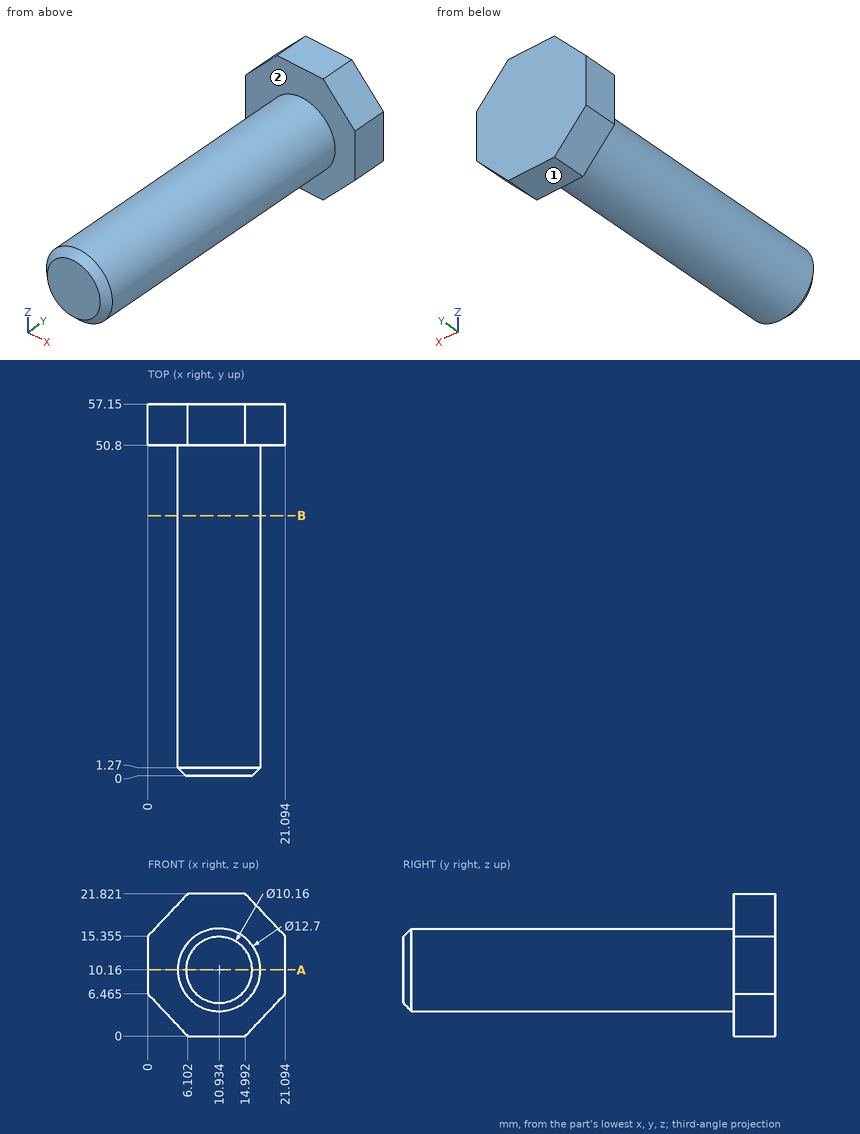
Answer from the drawing. Dimensions are ordinates in mm from the lowest x, y and z of the part. A direction names the side the tool comes from. Give positions to 0.01 mm unless a question says otherwise; leave off trailing zeros. Write each loop counter-clockwise with the first axis right and the second up, starting at its lowest first coordinate (ties: lowest second). Pieces come first, ordered by that corner, then holes.
1) Find the intervals of material crossed by L1, parallel to Y at x = 13.25, z = 16.25; L2, parallel to Z at x = 14.75, y = 35.5 (1 decimal); L3, parallel to X at y = 11, z = 10.25 (1 decimal), in increasing order.
2) Section A-A (z = 10.16) is taken. Write down the section's boundary in (x, y).
3) A tool of negligible diameter and unlimited length cuts with its end or side. For the marked faces 1 and 2, from which of +Z, -Z, +X, -X, +Y, -Y can it reach the whole face along a straight path? Write none if from no direction.
4) Given P1, Ø6, axis at x = 7, y = 26, coming from the +Z side; P2, Ø3, axis at x = 11.5, y = 32.5, coming from the +Z side; P3, Ø3, axis at y = 43, z = 8, coming from the -X side; P4, Ø8, axis at x = 11.5, z = 11.5, coming from the -Y side, each flat-ended and moving along its own axis, determine where each tip first touches the part or whether it passes through.
5) Section B-B (y = 40) is taken. Write down the section's boundary in (x, z).
Response:
1. L1: y = 50.8 to 57.15
1. L2: z = 5.1 to 15.2
1. L3: x = 4.6 to 17.3
2. outline: (0, 50.8) - (4.58, 50.8) - (4.58, 1.27) - (5.85, 0) - (16.01, 0) - (17.28, 1.27) - (17.28, 50.8) - (21.09, 50.8) - (21.09, 57.15) - (0, 57.15) - close
3. face 1: -Z, +X, -X, +Y, -Y
3. face 2: -Y
4. P1: stops at z = 16.44
4. P2: stops at z = 16.51
4. P3: stops at x = 4.62
4. P4: stops at y = 0
5. outline: circle Ø12.7 at (10.93, 10.16)
